Model file for the job. Use its own axes, mm. A direction names the side the tool comes from. Coordinates: 2 decimals unless noted, no trailing zeros. Order: outer loops, then holes, each group sorted by start corner. A loop starts at its lowest first (then second) coordinate and runs counter-clockwise, first axis right, second up. Notation, with made-up numbers: (-1, 86) -> (27, 86) arc R25 ccw to (27, 115) -> close; hole circle Ø6 at (-15, 35). An arc over 180 degrees is marked (long way). Return JSON: item names as keys, results as strings. Group by question number.
1) Which spindle directions (+Z, -Z, +X, -X, +Y, -Y) get a long thin tool onto all of the face, cutting with end or side? Do faces 5 (the flat face through (3, -13, 46.477)), 6 (the flat face through (-48, -13, 23.686)), 7 (the flat face through (-48, -50.8, 5)), 8 (the flat face through (-14, 0, -9)), 9 (the flat face through (-9.865, -13, 22)). Say none if no direction does.
2) Cut at D-D (x = -46). Write the cut outline in (y, z).
3) Cut at B-B (y = -65). Write the cut outline in (x, z).
4) Cut at C-C (z = 36.5). Write the cut outline in (x, y), and give its area (3 significant figures).
5) Flat gauge pins, fed straight in: pin 1 (12.5 mm diameter, centred on x = -53.5, y = -17.5, fed in from +Z); pin 2 (7.5 mm diameter, centred on y = -14.5, z = 30, fed in from -X); pin 3 (7.5 mm diameter, centred on x = -44.5, y = -69, fed in from +Z). Where does each tip first touch, or does it go through?
6) Probe line 1 (Y direction, x = 1, z = 20); line 2 (X direction, y = -8.5, z = 17); line 3 (Z direction, x = -13, y = -52). List the from-to ranges inside material, lowest first.
7) Pull direction X, two halves, no side cores. Call faces 1 (the flat face through (-60.665, -38, -9)), 2 (the flat face through (-48, -63, 10.986)), 3 (the flat face through (15.535, -39, -6)), 4 (the flat face through (-35.265, -13, 11)): +X half, -X half, draft (parallel to the pull), parting line (faces both ways), or undercut.
8) Cut at A-A (z = 2). Write the cut outline in (x, y).
from build123d import *

# Parameters (mm, degrees)
F1_DEPTH  = 76.2
F2_W      = 25.4
F2_H      = 25.4
F3_DEPTH  = 38.1
F4_W      = 25.4
F4_H      = 25.4
F5_DEPTH  = 12.7
F6_DEPTH  = 12.7
F7_W      = 25.4
F7_H      = 25.4
F8_DEPTH  = 35.56
F9_DEPTH  = 25.4
F10_DEPTH = 12.7


with BuildPart() as f1:
    # F0 (on Front) → F1 (new body)
    with BuildSketch(Plane.XZ):
        Polygon((-60.6652237475, 10.9855490685), (-60.6652237475, -29.7227894413), (15.5347762525, -29.7227894413), (15.5347762525, 33.7772105587), (-9.8652237475, 33.7772105587), (-9.8652237475, -1.7144509315), (-35.2652237475, -1.7144509315), (-35.2652237475, 10.9855490685), align=None)
    extrude(amount=F1_DEPTH)

    # F2 (on face) → F3 (join)
    with BuildSketch(Plane.XY.offset(33.7772105587)):
        with Locations((2.8347762525, -38.1)):
            Rectangle(F2_W, F2_H)
    extrude(amount=-F3_DEPTH)

    # F4 (on face) → F5 (cut)
    with BuildSketch(Plane.XY.offset(10.9855490685)):
        with Locations((-47.9652237475, -38.1)):
            Rectangle(F4_W, F4_H)
    extrude(amount=-F5_DEPTH, mode=Mode.SUBTRACT)

    # F6 (add): a face of the model
    f6_faces = [f1.faces().sort_by_distance(p)[0] for p in [
        (-47.9652237475, -12.7, 10.9855490685),
    ]]
    extrude(f6_faces, amount=F6_DEPTH)

    # F7 (on face) → F8 (cut)
    with BuildSketch(Plane.XY.offset(33.7772105587)):
        with Locations((2.8347762525, -38.1)):
            Rectangle(F7_W, F7_H)
    extrude(amount=-F8_DEPTH, mode=Mode.SUBTRACT)

    # F9 (add): a face of the model
    f9_faces = [f1.faces().sort_by_distance(p)[0] for p in [
        (2.8347762525, -63.5, 33.7772105587),
    ]]
    extrude(f9_faces, amount=F9_DEPTH)

    # F10 (add): a face of the model
    f10_faces = [f1.faces().sort_by_distance(p)[0] for p in [
        (2.8347762525, -12.7, 33.7772105587),
    ]]
    extrude(f10_faces, amount=F10_DEPTH)


solid = f1.part
Answers below:
{
 "1": {"face 5": "+Z, +X, -X, +Y", "face 6": "+Z, -X, +Y, -Y", "face 7": "+Z, +X, -X", "face 8": "+Z, -Z, +X, -X, +Y", "face 9": "+Z, +Y, -Y"},
 "2": {"outline": "(-76.2, -29.72) -> (0, -29.72) -> (0, 23.69) -> (-25.4, 23.69) -> (-25.4, -1.71) -> (-50.8, -1.71) -> (-50.8, 10.99) -> (-76.2, 10.99) -> close"},
 "3": {"outline": "(-60.67, -29.72) -> (15.53, -29.72) -> (15.53, 59.18) -> (-9.87, 59.18) -> (-9.87, -1.71) -> (-35.27, -1.71) -> (-35.27, 10.99) -> (-60.67, 10.99) -> close"},
 "4": {"outline": "(-9.87, -76.2) -> (15.53, -76.2) -> (15.53, -50.8) -> (-9.87, -50.8) -> close; (-9.87, -25.4) -> (15.53, -25.4) -> (15.53, 0) -> (-9.87, 0) -> close", "area": "1,290 mm^2"},
 "5": {"pin 1": "stops at z = 23.69", "pin 2": "stops at x = -9.87", "pin 3": "stops at z = 10.99"},
 "6": {"line 1": "y = -76.2 to -50.8, -25.4 to 0", "line 2": "x = -60.67 to -35.27, -9.87 to 15.53", "line 3": "z = -29.72 to -1.71"},
 "7": {"face 1": "-X half", "face 2": "draft", "face 3": "+X half", "face 4": "undercut"},
 "8": {"outline": "(-60.67, -76.2) -> (-35.27, -76.2) -> (-35.27, -50.8) -> (-60.67, -50.8) -> close; (-60.67, -25.4) -> (-35.27, -25.4) -> (-35.27, 0) -> (-60.67, 0) -> close; (-9.87, -76.2) -> (15.53, -76.2) -> (15.53, -50.8) -> (-9.87, -50.8) -> close; (-9.87, -25.4) -> (15.53, -25.4) -> (15.53, 0) -> (-9.87, 0) -> close"}
}
